Can you work these out from the model? Positions are in its coordinate system, mm. Coordinates: 2 decimals unless noted, no trailing zeros. Loops run counter-clockwise (first coordinate to the right, second up) from the corner with the lowest first, then second, coordinate; pieces in that order, holes last.
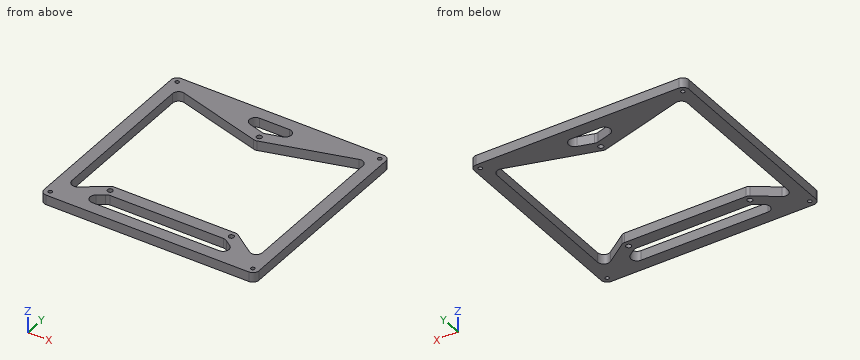
```python
from build123d import *

# Parameters (mm, degrees)
BOSS_EXTRU_1_DEPTH = 8
D_GAGEMENT_M31_D   = 3.2
D_GAGEMENT_M41_D   = 4.3


with BuildPart() as part:
    # Esquisse1 → Boss.-Extru.1 (new body)
    with BuildSketch(Plane.XY):
        with BuildLine():
            Line((-83.5, -84), (83.5, -84))
            ThreePointArc((83.5, -84), (87.035533906, -82.535533906), (88.5, -79))
            Line((88.5, -79), (88.5, 79))
            ThreePointArc((88.5, 79), (87.035533906, 82.535533906), (83.5, 84))
            Line((83.5, 84), (-83.5, 84))
            ThreePointArc((-83.5, 84), (-87.035533906, 82.535533906), (-88.5, 79))
            Line((-88.5, 79), (-88.5, -79))
            ThreePointArc((-88.5, -79), (-87.035533906, -82.535533906), (-83.5, -84))
        make_face()
        with BuildLine():
            Line((-52.904447079, -51.023190589), (-70.595552921, -63.648248646))
            ThreePointArc((-70.595552921, -63.648248646), (-75.788860481, -64.02368409), (-78.5, -59.578336218))
            Line((-78.5, -59.578336218), (-78.5, 65.735103055))
            ThreePointArc((-78.5, 65.735103055), (-76.509878124, 69.727675368), (-72.123746529, 70.541965481))
            Line((-72.123746529, 70.541965481), (-1.376253471, 50.286240591))
            ThreePointArc((-1.376253471, 50.286240591), (0, 50.093103017), (1.376253471, 50.286240591))
            Line((1.376253471, 50.286240591), (72.123746529, 70.541965481))
            ThreePointArc((72.123746529, 70.541965481), (76.509878124, 69.727675368), (78.5, 65.735103055))
            Line((78.5, 65.735103055), (78.5, -59.578336218))
            ThreePointArc((78.5, -59.578336218), (75.788860481, -64.02368409), (70.595552921, -63.648248646))
            Line((70.595552921, -63.648248646), (52.904447079, -51.023190589))
            ThreePointArc((52.904447079, -51.023190589), (51.524866857, -50.331298625), (50, -50.093103017))
            Line((50, -50.093103017), (-50, -50.093103017))
            ThreePointArc((-50, -50.093103017), (-51.524866857, -50.331298625), (-52.904447079, -51.023190589))
        make_face(mode=Mode.SUBTRACT)
        with BuildLine():
            Line((-49.702159182, -61.023190589), (-55.176773853, -64.930087573))
            ThreePointArc((-55.176773853, -64.930087573), (-57.034131166, -70.524866857), (-52.272326774, -74))
            Line((-52.272326774, -74), (52.272326774, -74))
            ThreePointArc((52.272326774, -74), (57.034131166, -70.524866857), (55.176773853, -64.930087573))
            Line((55.176773853, -64.930087573), (49.702159182, -61.023190589))
            ThreePointArc((49.702159182, -61.023190589), (48.322578961, -60.331298625), (46.797712104, -60.093103017))
            Line((46.797712104, -60.093103017), (-46.797712104, -60.093103017))
            ThreePointArc((-46.797712104, -60.093103017), (-48.322578961, -60.331298625), (-49.702159182, -61.023190589))
        make_face(mode=Mode.SUBTRACT)
        with BuildLine():
            Line((-13.618577234, 64.193137574), (-1.376253471, 60.6880361))
            ThreePointArc((-1.376253471, 60.6880361), (0, 60.494898526), (1.376253471, 60.6880361))
            Line((1.376253471, 60.6880361), (13.618577234, 64.193137574))
            ThreePointArc((13.618577234, 64.193137574), (17.193803952, 69.694869725), (12.242323763, 74))
            Line((12.242323763, 74), (-12.242323763, 74))
            ThreePointArc((-12.242323763, 74), (-17.193803952, 69.694869725), (-13.618577234, 64.193137574))
        make_face(mode=Mode.SUBTRACT)
    extrude(amount=BOSS_EXTRU_1_DEPTH)

    # Dégagement M31 (through all)
    with Locations(Plane.XY.offset(8)):
        with Locations((-83.5, 79), (-83.5, -79), (83.5, -79), (83.5, 79)):
            Hole(D_GAGEMENT_M31_D / 2)

    # Dégagement M41 (through all)
    with Locations(Plane.XY.offset(8)):
        with Locations((-50, -55.093103017), (50, -55.093103017), (0, 55.093103017)):
            Hole(D_GAGEMENT_M41_D / 2)


solid = part.part
```
(1) I'm going to push a flat-ended pin straight in: pin 1 (1.9 mm diameter, centred on x = 83.5, y = 79, fed in from +Z). Where does the tip first touch, or does it pass through?
Check values:
pin 1: passes through
(2) If I drill on probe 1 along X at (y, z) = (79, 2.5); probe 2 along Y at (x, z) = (83.5, 4.5); probe 3 along X at (y, z) = (-40, 2.5), over which ranges is the centre line in solid material (lowest first)?
Check values:
probe 1: x = -88.5 to -85.1, -81.9 to 81.9, 85.1 to 88.5
probe 2: y = -84 to -80.6, -77.4 to 77.4, 80.6 to 84
probe 3: x = -88.5 to -78.5, 78.5 to 88.5
(3) I want a section at C-C on z = 2. State how many separate pieces and enclosed holes the cut face has, then the cut area to 3 significant figures.
Check values:
separate pieces: 1
enclosed holes: 10
area: 9,830 mm2
(4) I want a section at B-B on x = 21.5. Write out the boundary of the cut face in (y, z).
Check values:
outline: (-84, 0) - (-74, 0) - (-74, 8) - (-84, 8) - close; (-60.09, 0) - (-50.09, 0) - (-50.09, 8) - (-60.09, 8) - close; (56.05, 0) - (84, 0) - (84, 8) - (56.05, 8) - close
(5) I want a section at A-A on y = -15.5. Write out the boundary of the cut face in (x, z), then the cut area to 3 significant figures.
Check values:
outline: (-88.5, 0) - (-78.5, 0) - (-78.5, 8) - (-88.5, 8) - close; (78.5, 0) - (88.5, 0) - (88.5, 8) - (78.5, 8) - close
area: 160 mm2
